Can you work these out from the model? Positions are in its coordinate system, mm. A direction names the side the tool comes from. Give positions to 0.01 mm unless a question says otherwise; leave off trailing zeros. Write each loop counter-clockwise with the first axis right and the second up, starting at its lowest first coordinate (ties: lowest second). Pieces come first, ordered by that corner, then holes.
from build123d import *

# Parameters (mm, degrees)
SKETCH001_W          = 15
SKETCH001_H          = 28.85
PAD_DEPTH            = 5.6
SKETCH002_R          = 2.25
SKETCH002_W          = 2.3
SKETCH002_H          = 6.2
SKETCH002_W_2        = 2.4
SKETCH002_H_2        = 7.3
PAD001_DEPTH         = 1
SKETCH010_W          = 2.3
SKETCH010_H          = 6.2
SKETCH010_W_2        = 2.4
SKETCH010_H_2        = 5.4
PAD004_DEPTH         = 2.55
SKETCH003_R          = 1.6
PAD002_DEPTH         = 1.55
PAD006_DEPTH         = 6.2
PAD005_DEPTH         = 5.4
POCKET_DEPTH         = 0.9
SKETCH013_W          = 10.4
SKETCH013_H          = 6.2
POCKET003_DEPTH      = 1.2
CHAMFER_SIZE2        = 1.5
CHAMFER_SIZE         = 0.8
FILLET_R             = 0.4
SKETCH009_R          = 1.6
POCKET002_DEPTH      = 7.501
POCKET002_DEPTH_BACK = 7.501


with BuildPart() as part:
    # Sketch001 → Pad (new body)
    with BuildSketch(Plane.XY):
        with Locations((0, -4.925)):
            Rectangle(SKETCH001_W, SKETCH001_H)
    extrude(amount=PAD_DEPTH)

    # Sketch002 → Pad001 (join)
    with BuildSketch(Plane.XY.offset(5.6)):
        with Locations((-5.25, 0)):
            Circle(SKETCH002_R)
        with Locations((5.25, 0)):
            Circle(SKETCH002_R)
        with Locations((-6.35, 6.4)):
            Rectangle(SKETCH002_W, SKETCH002_H)
        with Locations((6.35, 6.4)):
            Rectangle(SKETCH002_W, SKETCH002_H)
        with Locations((-6.3, -15.7)):
            Rectangle(SKETCH002_W_2, SKETCH002_H_2)
        with Locations((6.3, -15.7)):
            Rectangle(SKETCH002_W_2, SKETCH002_H_2)
    extrude(amount=PAD001_DEPTH)

    # Sketch010 → Pad004 (join)
    with BuildSketch(Plane.XY.offset(6.6)):
        with Locations((-6.35, 6.4)):
            Rectangle(SKETCH010_W, SKETCH010_H)
        with Locations((6.35, 6.4)):
            Rectangle(SKETCH010_W, SKETCH010_H)
        with Locations((6.3, -14.75)):
            Rectangle(SKETCH010_W_2, SKETCH010_H_2)
        with Locations((-6.3, -14.75)):
            Rectangle(SKETCH010_W_2, SKETCH010_H_2)
    extrude(amount=PAD004_DEPTH)

    # Sketch003 → Pad002 (join)
    with BuildSketch(Plane.XY.offset(6.6)):
        with Locations((-5.25, 0)):
            Circle(SKETCH003_R)
        with Locations((5.25, 0)):
            Circle(SKETCH003_R)
    extrude(amount=PAD002_DEPTH)

    # Sketch012 (on DatumPlane) → Pad006 (join)
    with BuildSketch(Plane(origin=(5.2, 9.5, 0), x_dir=(1, 0, 0), z_dir=(0, -1, 0))):
        Polygon((0, 8.15), (0, 9.15), (-0.15, 8.236603), align=None)
        Polygon((-10.4, 8.15), (-10.4, 9.15), (-10.25, 8.236603), align=None)
    extrude(amount=PAD006_DEPTH)

    # Sketch011 (on DatumPlane) → Pad005 (join)
    with BuildSketch(Plane(origin=(-5.1, -12.05, 0), x_dir=(-1, 0, 0), z_dir=(0, 1, 0))):
        Polygon((0, 8.15), (-0.15, 8.236603), (0, 9.15), align=None)
        Polygon((-10.2, 8.15), (-10.2, 9.15), (-10.05, 8.236603), align=None)
    extrude(amount=-PAD005_DEPTH)

    # Sketch004 → Pocket (cut)
    with BuildSketch(Plane.XY.offset(5.6)):
        with BuildLine():
            ThreePointArc((-5.1, -2.244994), (-3.000557, 0.050049), (-5.2, 2.249444))
            Line((-5.2, 9.5), (-5.2, 2.249444))
            Line((-5.2, 9.5), (5.2, 9.5))
            Line((5.2, 9.5), (5.2, 2.249444))
            ThreePointArc((5.2, 2.249444), (3.000557, 0.050049), (5.1, -2.244994))
            Line((5.1, -19.35), (5.1, -2.244994))
            Line((-5.1, -19.35), (5.1, -19.35))
            Line((-5.1, -19.35), (-5.1, -2.244994))
        make_face()
    extrude(amount=-POCKET_DEPTH, mode=Mode.SUBTRACT)

    # Sketch013 → Pocket003 (cut)
    with BuildSketch(Plane.XY.offset(5.6)):
        with Locations((0, 6.4)):
            Rectangle(SKETCH013_W, SKETCH013_H)
    extrude(amount=-POCKET003_DEPTH, mode=Mode.SUBTRACT)

    # Chamfer
    chamfer_edges = [part.edges().sort_by_distance(p)[0] for p in [
        (0, -19.35, 4.7),
    ]]
    chamfer_side = part.faces().sort_by_distance((0, -19.35, 2.727995))[0]
    chamfer(chamfer_edges, length=CHAMFER_SIZE, length2=CHAMFER_SIZE2, reference=chamfer_side)

    # Fillet
    fillet_edges = [part.edges().sort_by_distance(p)[0] for p in [
        (-5.025, -17.45, 8.693301),
        (-5.1, -17.45, 7.375),
        (-5.025, -17.45, 8.193301),
        (5.1, -17.45, 7.375),
        (5.025, -17.45, 8.193301),
        (5.025, -17.45, 8.693301),
        (-5.2, 3.3, 6.875),
        (-5.125, 3.3, 8.193301),
        (-5.125, 3.3, 8.693301),
        (5.2, 3.3, 6.875),
        (5.125, 3.3, 8.193301),
        (5.125, 3.3, 8.693301),
        (5.125, 9.5, 8.693301),
        (5.125, 9.5, 8.193301),
        (5.2, 9.5, 6.275),
        (-5.125, 9.5, 8.693301),
        (-5.125, 9.5, 8.193301),
        (-5.2, 9.5, 6.275),
        (-5.1, -12.05, 6.875),
        (-5.025, -12.05, 8.193301),
        (-5.025, -12.05, 8.693301),
        (5.025, -12.05, 8.693301),
        (5.025, -12.05, 8.193301),
        (5.1, -12.05, 6.875),
        (-6.85, 0, 8.15),
        (3.65, 0, 8.15),
        (5.2, 6.4, 9.15),
        (5.1, -14.75, 9.15),
        (-5.1, -14.75, 9.15),
        (-5.2, 6.4, 9.15),
        (6.35, 9.5, 9.15),
        (6.35, 3.3, 9.15),
        (7.5, 6.4, 9.15),
        (6.3, -12.05, 9.15),
        (7.5, -14.75, 9.15),
        (6.3, -17.45, 9.15),
        (-6.35, 9.5, 9.15),
        (-7.5, 6.4, 9.15),
        (-6.35, 3.3, 9.15),
        (-7.5, -14.75, 9.15),
        (-6.3, -17.45, 9.15),
        (-7.5, -17.45, 7.875),
        (-6.3, -12.05, 9.15),
        (-7.5, -12.05, 7.375),
        (7.5, -12.05, 7.375),
        (-7.5, 3.3, 7.375),
        (7.5, -17.45, 7.875),
        (7.5, 3.3, 7.375),
        (-7.5, -19.35, 3.3),
        (7.5, -19.35, 3.3),
        (7.5, 9.5, 4.575),
        (-7.5, 9.5, 4.575),
        (-5.1, -19.35, 5.65),
        (5.1, -19.35, 5.65),
    ]]
    fillet(fillet_edges, radius=FILLET_R)

    # Sketch009 → Pocket002 (cut, two sides)
    with BuildSketch(Plane.YZ) as pocket002_sk:
        with Locations((-1.4, 2.8)):
            Circle(SKETCH009_R)
    extrude(amount=-POCKET002_DEPTH, mode=Mode.SUBTRACT)
    extrude(pocket002_sk.sketch, amount=POCKET002_DEPTH_BACK, mode=Mode.SUBTRACT)


solid = part.part
(1) If we mould it in two halves opening along X, with no side actions, what happens to faces 5 (the face through (-5.1, -13, 6)), 6 (the face through (7.5, -5, 3)), 7 (the face through (0, -5, 0)), 8 (the face through (-6.85, 0.07, 7.17))? For each: +X half, -X half, draft (parallel to the pull), parting line (faces both ways), or undercut.
Returned:
face 5: undercut
face 6: +X half
face 7: draft
face 8: undercut
(2) If I drill on L1, parallel to X at y = 7.25, z = 7; L2, parallel to X at y = -13.75, z = 7.5; L3, parallel to Y at x = 5.25, z = 2.8, over which ranges is the centre line in solid material (lowest first)?
Returned:
L1: x = -7.5 to -5.2, 5.2 to 7.5
L2: x = -7.5 to -5.1, 5.1 to 7.5
L3: y = -19.35 to -3, 0.2 to 9.5
(3) Imagine slicing it at D-D, the plane y = 7.5. Write out the boundary of the cut face in (x, z).
Returned:
outline: (-7.5, 0) - (7.5, 0) - (7.5, 8.75) arc R0.4 ccw to (7.1, 9.15) - (5.54, 9.15) arc R0.4 ccw to (5.14, 8.81) - (5.05, 8.24) - (5.2, 8.15) - (5.2, 4.4) - (-5.2, 4.4) - (-5.2, 8.15) - (-5.05, 8.24) - (-5.14, 8.81) arc R0.4 ccw to (-5.54, 9.15) - (-7.1, 9.15) arc R0.4 ccw to (-7.5, 8.75) - close
(4) For faces 1 (the face through (-0.1, -18.6, 4.3)), 2 (the face through (3.65, 0.07, 7.17)), 3 (the face through (6, -12.05, 7)), 4 (the face through (-6, -17.45, 8)), which set-ups out of +Z, -Z, +X, -X, +Y, -Y let a thin tool reach every point of the face, with its end or its side?
Returned:
face 1: +Z, -Y
face 2: +Z
face 3: +Z, +X, -X
face 4: +Z, +X, -X, -Y
(5) Imagine slicing it at C-C, the plane x = -2.25. Write out the boundary of the cut face in (y, z).
Returned:
outline: (-19.35, 0) - (9.5, 0) - (9.5, 4.4) - (3.3, 4.4) - (3.3, 4.7) - (-17.85, 4.7) - (-19.35, 3.9) - close; hole circle Ø3.2 at (-1.4, 2.8)
(6) Imagine slicing it at B-B, the plane y = -11.25. Write out the boundary of the cut face in (x, z), plus the area to 3 significant figures.
Returned:
outline: (-7.5, 0) - (7.5, 0) - (7.5, 5.6) - (5.1, 5.6) - (5.1, 4.7) - (-5.1, 4.7) - (-5.1, 5.6) - (-7.5, 5.6) - close
area: 74.8 mm2
(7) Imagine slicing it at A-A, the plane z = 2.8. Write out the boundary of the cut face in (x, y), plus the area to 3 significant figures.
Returned:
outline: (-7.5, -18.95) arc R0.4 ccw to (-7.1, -19.35) - (7.1, -19.35) arc R0.4 ccw to (7.5, -18.95) - (7.5, -3) - (-7.5, -3) - close; (-7.5, 0.2) - (7.5, 0.2) - (7.5, 9.1) arc R0.4 ccw to (7.1, 9.5) - (-7.1, 9.5) arc R0.4 ccw to (-7.5, 9.1) - close
area: 385 mm2
(8) Will these pins go through, and if not, where does the flat tip stop? P1, Ø3.5, axis at x = 4.5, y = 0.5, coming from the +Z side; P2, Ø1.2, axis at x = -7, y = 2, coming from the +Z side; P3, Ø0.9, axis at x = 6.5, z = 8, coming from the -Y side.
Returned:
P1: stops at z = 8.15
P2: stops at z = 6.6
P3: stops at y = -17.45
